Source: CAD feature listing. Evaluate the final solid. Frame: model axes, mm. Give positions to 0.01 mm unless a question says otherwise; leave off trailing zeros. Write each loop counter-clockwise with the first axis right and the second up, starting at its lowest first coordinate (ties: lowest second). Pieces come first, ordered by that corner, then holes.
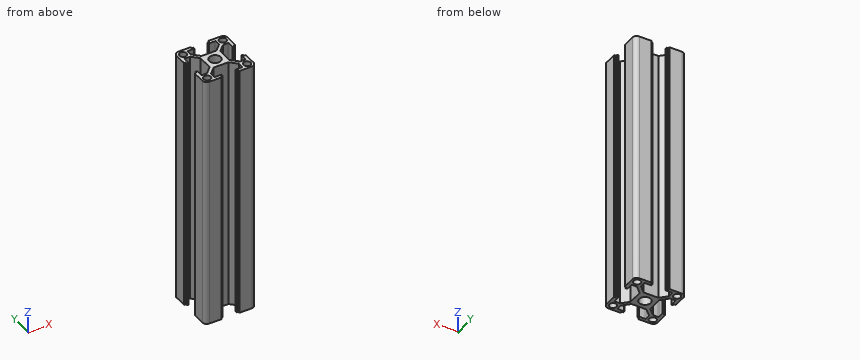
```python
from build123d import *

# Parameters (mm, degrees)
CROQUIS1_R              = 2.1
CROQUIS1_R_2            = 3.4
SALIENTE_EXTRUIR1_DEPTH = 400
CROQUIS2_W              = 39.308064919
CROQUIS2_H              = 32.219725343
CORTAR_EXTRUIR1_DEPTH   = 250


with BuildPart() as part:
    # Croquis1 → Saliente-Extruir1 (new body)
    with BuildSketch(Plane(origin=(0, 0, -50), x_dir=(-1, 0, 0), z_dir=(0, 0, -1))):
        with BuildLine():
            Line((14.7, -5.1), (14.3, -5.1))
            ThreePointArc((14.3, -5.1), (14.087867966, -5.012132034), (14, -4.8))
            Line((14, -4.8), (14, -4.4))
            ThreePointArc((14, -4.4), (13.912132034, -4.187867966), (13.7, -4.1))
            Line((13.7, -4.1), (13.3, -4.1))
            ThreePointArc((13.3, -4.1), (13.087867966, -4.187867966), (13, -4.4))
            Line((13, -4.4), (13, -7.95))
            ThreePointArc((13, -7.95), (12.912132034, -8.162132034), (12.7, -8.25))
            Line((12.7, -8.25), (9.789264108, -8.25))
            ThreePointArc((9.789264108, -8.25), (9.674477865, -8.22717164), (9.577160832, -8.162160788))
            Line((9.577160832, -8.162160788), (5.887896723, -4.473896751))
            ThreePointArc((5.887896723, -4.473896751), (5.822843922, -4.376559778), (5.8, -4.261735963))
            Line((5.8, -4.261735963), (5.8, 4.260735931))
            ThreePointArc((5.8, 4.260735931), (5.82283614, 4.375540961), (5.887867966, 4.472867966))
            Line((5.887867966, 4.472867966), (9.577132034, 8.162132034))
            ThreePointArc((9.577132034, 8.162132034), (9.674459039, 8.22716386), (9.789264069, 8.25))
            Line((9.789264069, 8.25), (12.7, 8.25))
            ThreePointArc((12.7, 8.25), (12.912132034, 8.162132034), (13, 7.95))
            Line((13, 7.95), (13, 4.4))
            ThreePointArc((13, 4.4), (13.087867966, 4.187867966), (13.3, 4.1))
            Line((13.3, 4.1), (13.7, 4.1))
            ThreePointArc((13.7, 4.1), (13.912132034, 4.187867966), (14, 4.4))
            Line((14, 4.4), (14, 4.8))
            ThreePointArc((14, 4.8), (14.087867966, 5.012132034), (14.3, 5.1))
            Line((14.3, 5.1), (14.7, 5.1))
            ThreePointArc((14.7, 5.1), (14.912132034, 5.187867966), (15, 5.4))
            Line((15, 5.4), (15, 12.5))
            ThreePointArc((15, 12.5), (14.267766953, 14.267766953), (12.5, 15))
            Line((12.5, 15), (5.4, 15))
            ThreePointArc((5.4, 15), (5.187867966, 14.912132034), (5.1, 14.7))
            Line((5.1, 14.7), (5.1, 14.3))
            ThreePointArc((5.1, 14.3), (5.012132034, 14.087867966), (4.8, 14))
            Line((4.8, 14), (4.4, 14))
            ThreePointArc((4.4, 14), (4.187867966, 13.912132034), (4.1, 13.7))
            Line((4.1, 13.7), (4.1, 13.3))
            ThreePointArc((4.1, 13.3), (4.187867966, 13.087867966), (4.4, 13))
            Line((4.4, 13), (7.95, 13))
            ThreePointArc((7.95, 13), (8.162132034, 12.912132034), (8.25, 12.7))
            Line((8.25, 12.7), (8.25, 9.788264069))
            ThreePointArc((8.25, 9.788264069), (8.22716386, 9.673459039), (8.162132034, 9.576132034))
            Line((8.162132034, 9.576132034), (4.473867966, 5.887867966))
            ThreePointArc((4.473867966, 5.887867966), (4.376540961, 5.82283614), (4.261735931, 5.8))
            Line((4.261735931, 5.8), (-4.260735892, 5.8))
            ThreePointArc((-4.260735892, 5.8), (-4.375522135, 5.82282836), (-4.472839168, 5.887839212))
            Line((-4.472839168, 5.887839212), (-8.162103277, 9.576103249))
            ThreePointArc((-8.162103277, 9.576103249), (-8.227156078, 9.673440222), (-8.25, 9.788264037))
            Line((-8.25, 9.788264037), (-8.25, 12.7))
            ThreePointArc((-8.25, 12.7), (-8.162132034, 12.912132034), (-7.95, 13))
            Line((-7.95, 13), (-4.4, 13))
            ThreePointArc((-4.4, 13), (-4.187867966, 13.087867966), (-4.1, 13.3))
            Line((-4.1, 13.3), (-4.1, 13.7))
            ThreePointArc((-4.1, 13.7), (-4.187867966, 13.912132034), (-4.4, 14))
            Line((-4.4, 14), (-4.8, 14))
            ThreePointArc((-4.8, 14), (-5.012132034, 14.087867966), (-5.1, 14.3))
            Line((-5.1, 14.3), (-5.1, 14.7))
            ThreePointArc((-5.1, 14.7), (-5.187867966, 14.912132034), (-5.4, 15))
            Line((-5.4, 15), (-12.5, 15))
            ThreePointArc((-12.5, 15), (-14.267766953, 14.267766953), (-15, 12.5))
            Line((-15, 12.5), (-15, 5.4))
            ThreePointArc((-15, 5.4), (-14.912132034, 5.187867966), (-14.7, 5.1))
            Line((-14.7, 5.1), (-14.3, 5.1))
            ThreePointArc((-14.3, 5.1), (-14.087867966, 5.012132034), (-14, 4.8))
            Line((-14, 4.8), (-14, 4.4))
            ThreePointArc((-14, 4.4), (-13.912132034, 4.187867966), (-13.7, 4.1))
            Line((-13.7, 4.1), (-13.3, 4.1))
            ThreePointArc((-13.3, 4.1), (-13.087867966, 4.187867966), (-13, 4.4))
            Line((-13, 4.4), (-13, 7.95))
            ThreePointArc((-13, 7.95), (-12.912132034, 8.162132034), (-12.7, 8.25))
            Line((-12.7, 8.25), (-9.788264037, 8.25))
            ThreePointArc((-9.788264037, 8.25), (-9.673440222, 8.227156078), (-9.576103249, 8.162103277))
            Line((-9.576103249, 8.162103277), (-5.887839212, 4.472839168))
            ThreePointArc((-5.887839212, 4.472839168), (-5.82282836, 4.375522135), (-5.8, 4.260735892))
            Line((-5.8, 4.260735892), (-5.8, -4.261735931))
            ThreePointArc((-5.8, -4.261735931), (-5.82283614, -4.376540961), (-5.887867966, -4.473867966))
            Line((-5.887867966, -4.473867966), (-9.576132034, -8.162132034))
            ThreePointArc((-9.576132034, -8.162132034), (-9.673459039, -8.22716386), (-9.788264069, -8.25))
            Line((-9.788264069, -8.25), (-12.7, -8.25))
            ThreePointArc((-12.7, -8.25), (-12.912132034, -8.162132034), (-13, -7.95))
            Line((-13, -7.95), (-13, -4.4))
            ThreePointArc((-13, -4.4), (-13.087867966, -4.187867966), (-13.3, -4.1))
            Line((-13.3, -4.1), (-13.7, -4.1))
            ThreePointArc((-13.7, -4.1), (-13.912132034, -4.187867966), (-14, -4.4))
            Line((-14, -4.4), (-14, -4.8))
            ThreePointArc((-14, -4.8), (-14.087867966, -5.012132034), (-14.3, -5.1))
            Line((-14.3, -5.1), (-14.7, -5.1))
            ThreePointArc((-14.7, -5.1), (-14.912132034, -5.187867966), (-15, -5.4))
            Line((-15, -5.4), (-15, -12.5))
            ThreePointArc((-15, -12.5), (-14.267766953, -14.267766953), (-12.5, -15))
            Line((-12.5, -15), (-5.4, -15))
            ThreePointArc((-5.4, -15), (-5.187867966, -14.912132034), (-5.1, -14.7))
            Line((-5.1, -14.7), (-5.1, -14.3))
            ThreePointArc((-5.1, -14.3), (-5.012132034, -14.087867966), (-4.8, -14))
            Line((-4.8, -14), (-4.4, -14))
            ThreePointArc((-4.4, -14), (-4.187867966, -13.912132034), (-4.1, -13.7))
            Line((-4.1, -13.7), (-4.1, -13.3))
            ThreePointArc((-4.1, -13.3), (-4.187867966, -13.087867966), (-4.4, -13))
            Line((-4.4, -13), (-7.95, -13))
            ThreePointArc((-7.95, -13), (-8.162132034, -12.912132034), (-8.25, -12.7))
            Line((-8.25, -12.7), (-8.25, -9.789264069))
            ThreePointArc((-8.25, -9.789264069), (-8.22716386, -9.674459039), (-8.162132034, -9.577132034))
            Line((-8.162132034, -9.577132034), (-4.472867966, -5.887867966))
            ThreePointArc((-4.472867966, -5.887867966), (-4.375540961, -5.82283614), (-4.260735931, -5.8))
            Line((-4.260735931, -5.8), (4.261735963, -5.8))
            ThreePointArc((4.261735963, -5.8), (4.376559778, -5.822843922), (4.473896751, -5.887896723))
            Line((4.473896751, -5.887896723), (8.162160788, -9.577160832))
            ThreePointArc((8.162160788, -9.577160832), (8.22717164, -9.674477865), (8.25, -9.789264108))
            Line((8.25, -9.789264108), (8.25, -12.7))
            ThreePointArc((8.25, -12.7), (8.162132034, -12.912132034), (7.95, -13))
            Line((7.95, -13), (4.4, -13))
            ThreePointArc((4.4, -13), (4.187867966, -13.087867966), (4.1, -13.3))
            Line((4.1, -13.3), (4.1, -13.7))
            ThreePointArc((4.1, -13.7), (4.187867966, -13.912132034), (4.4, -14))
            Line((4.4, -14), (4.8, -14))
            ThreePointArc((4.8, -14), (5.012132034, -14.087867966), (5.1, -14.3))
            Line((5.1, -14.3), (5.1, -14.7))
            ThreePointArc((5.1, -14.7), (5.187867966, -14.912132034), (5.4, -15))
            Line((5.4, -15), (12.5, -15))
            ThreePointArc((12.5, -15), (14.267766953, -14.267766953), (15, -12.5))
            Line((15, -12.5), (15, -5.4))
            ThreePointArc((15, -5.4), (14.912132034, -5.187867966), (14.7, -5.1))
        make_face()
        with Locations((-11.7, 11.7)):
            Circle(CROQUIS1_R, mode=Mode.SUBTRACT)
        with Locations((-11.7, -11.7)):
            Circle(CROQUIS1_R, mode=Mode.SUBTRACT)
        Circle(CROQUIS1_R_2, mode=Mode.SUBTRACT)
        with Locations((11.7, 11.7)):
            Circle(CROQUIS1_R, mode=Mode.SUBTRACT)
        with Locations((11.7, -11.7)):
            Circle(CROQUIS1_R, mode=Mode.SUBTRACT)
    extrude(amount=-SALIENTE_EXTRUIR1_DEPTH)

    # Croquis2 → Cortar-Extruir1 (cut)
    with BuildSketch(Plane(origin=(0, 0, -50), x_dir=(-1, 0, 0), z_dir=(0, 0, -1))):
        with Locations((0.664531836, 0.281922596)):
            Rectangle(CROQUIS2_W, CROQUIS2_H)
    extrude(amount=-CORTAR_EXTRUIR1_DEPTH, mode=Mode.SUBTRACT)


solid = part.part
```
1. Section query B-B (z = 331.5). Give the number of separate pieces and of enclosed holes in the cut face, plus the area to 3 significant figures.
2. Pin query (flat end, axial travel): P1, Ø4, axis at x = -1, z = 291.5, coming from the +Y side. Return the tip coordinate at first contact, or that it passes through.
3. Section query A-A (x = 0). Return loops of the section in (y, z).
4. Line query: probe 1 along X at (y, z) = (-11.5, 282.5); probe 2 along Y at (x, z) = (-11.7, 273); probe 3 along Y at (x, z) = (5.25, 241) (3 decimals). Output: solid intervals per line, ascending.
The answers:
1. separate pieces: 1
1. enclosed holes: 5
1. area: 314 mm2
2. P1: stops at y = 5.8
3. outline: (-5.8, 200) - (-3.4, 200) - (-3.4, 350) - (-5.8, 350) - close; (3.4, 200) - (5.8, 200) - (5.8, 350) - (3.4, 350) - close
4. probe 1: x = -15 to -13.79, -9.61 to -8.25, 8.25 to 9.61, 13.79 to 15
4. probe 2: y = -15 to -13.8, -9.6 to -8.25, 8.25 to 9.6, 13.8 to 15
4. probe 3: y = -14.96 to -13, -6.665 to 6.665, 13 to 14.96
